The model under review builds one solid part; all positions refer to its coordinate system, in mm. Round coordinates to 2 decimals unless told otherwise and drop trailing zeros. Order: outer loops, then holes, each group sorted by start corner. A loop starts at its lowest first (then second) coordinate and runs counter-clockwise, first axis right, second up. Notation, with made-up numbers: M 27,25.25 L 32,25.25 A34 cw 32,56.25 Z; hole C 7,68 d10. An arc over 180 degrees is marked long. Answer as CSV lines item,"result". Start each with the question number.
from build123d import *

# Parameters (mm, degrees)
SKETCH_1_R      = 1.354010502
EXTRUDE_1_DEPTH = 2


with BuildPart() as part:
    # 草图1 → 凸台-拉伸1 (new body)
    with BuildSketch(Plane.XY.offset(3)):
        with BuildLine():
            Line((55.860222099, 7.999), (-24.138320535, 7.999))
            ThreePointArc((-24.138320535, 7.999), (-26.96674766, 6.827427125), (-28.138320535, 3.999))
            ThreePointArc((-28.138320535, 3.999), (-26.966394209, 1.171219344), (-24.13832066, 0))
            Line((-24.13832066, 0), (55.860221974, 0))
            ThreePointArc((55.860221974, 0), (58.688649099, 1.171572875), (59.860221974, 4))
            ThreePointArc((59.860221974, 4), (58.688295648, 6.827780656), (55.860222099, 7.999))
        make_face()
        with Locations(Location((55.859733508, 3.999511534, 0), (0, 0, 180))):
            Circle(SKETCH_1_R, mode=Mode.SUBTRACT)
        with Locations(Location((-24.138809001, 3.998511534, 0), (0, 0, 180))):
            Circle(SKETCH_1_R, mode=Mode.SUBTRACT)
    extrude(amount=-EXTRUDE_1_DEPTH)


solid = part.part
Item 1: For pin 1 (4.5 mm diameter, centred on x = -24.14, y = 4, fed in from -Z), flat-tipped, find the tip position at first contact; note if it passes through.
Item 2: Wall thickness on probe 1 along X at (y, z) = (4.75, 2.05); probe 2 along X at (y, z) = (3.5, 2.8); probe 3 along X at (y, z) = (7.25, 1.5): over which ranges is each line inside the solid? List them lowest first. Write a range as [from, to].
Item 3: Consider section A-A (z = 1.95). State the section outline as (x, y) points, and give its area (3 significant figures).
Item 4: Consider section B-B (y = 7). State the section outline as (x, z) points.
Item 5: The part is to be moulded in two halves that separate along Y. For faces 1 (the flat face through (15, 0, 2)), 2 (the flat face through (15, 4, 3)), 3 (the cylindrical face through (-22.786, 3.939, 2.014)), 4 (the flat face through (16, 7.999, 2)), say which applies: +Y half, -Y half, draft (parallel to the pull), parting line (faces both ways), or undercut.
Reported:
1,pin 1,"stops at z = 1"
2,probe 1,"x = [-28.07, -25.27], [-23.01, 54.73], [56.99, 59.79]"
2,probe 2,"x = [-28.11, -25.4], [-22.88, 54.6], [57.12, 59.83]"
2,probe 3,"x = [-26.47, 58.19]"
3,outline,"M -28.14,4 A4 ccw -24.14,0 L 55.86,0 A4 ccw 59.86,4 A4 ccw 55.86,8 L -24.14,8 A4 ccw Z; hole C -24.14,4 d2.71; hole C 55.86,4 d2.71"
3,area,"679 mm²"
4,outline,"M -26.78,1 L 58.5,1 L 58.5,3 L -26.78,3 Z"
5,face 1,"-Y half"
5,face 2,"draft"
5,face 3,"undercut"
5,face 4,"+Y half"
